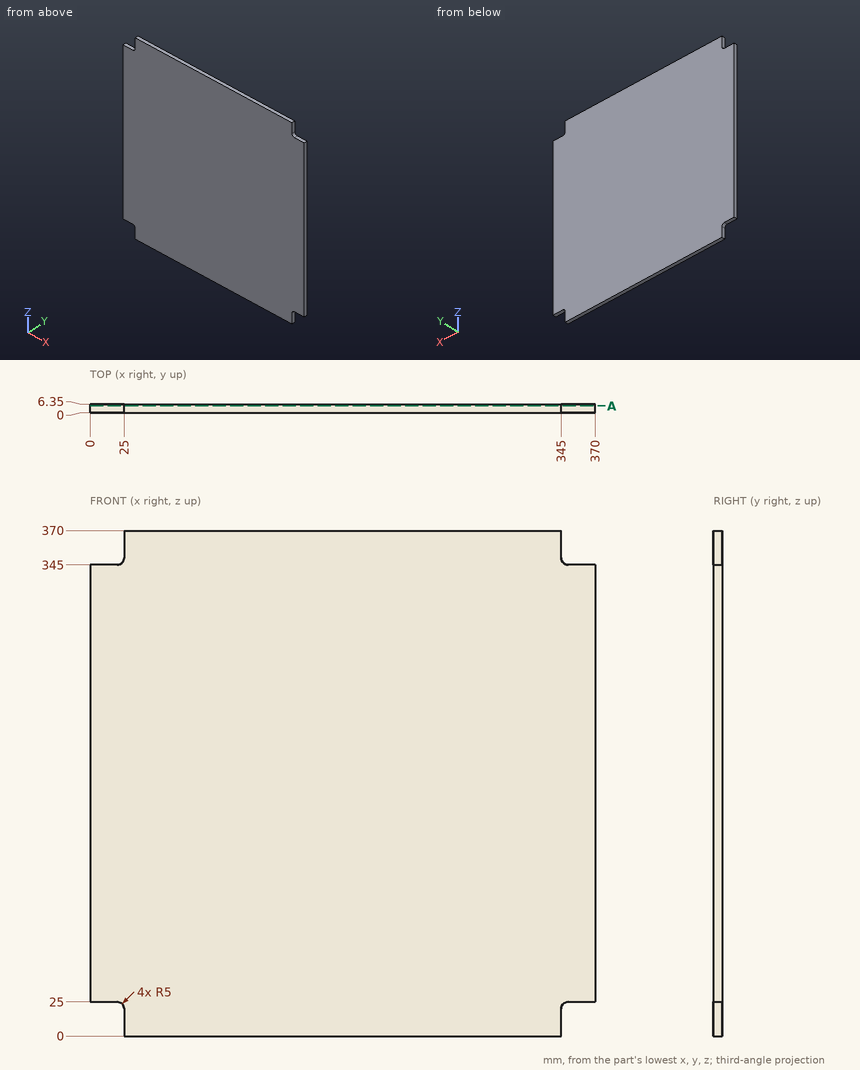
Part print with two shaded views. Sizes in mm from the minimum x, y, z corner. Give positions to 0.01 mm unless a question says otherwise; leave off trailing zeros. Order: outer loops, then holes, each group sorted by start corner. A loop starts at its lowest first (then second) coordinate and runs counter-clockwise, first axis right, second up.
1) Saw through at A-A, the plane y = 5. Write the cut outline in (x, z), then the cut area to 3 significant figures.
2) Wall check: probe 1 along Z at (x, y) = (18, 1.5); probe 2 along Z at (x, y) = (347.5, 0.75). Give the ranges that are in metal, low to high.
3) Pin check, flat tips, straight feed: pin 1 (1.9 mm diameter, centred on y = 3, z = 13.5, fed in from -X); pin 2 (3 mm diameter, centred on x = 8.5, y = 4, fed in from +Z); pin 3 (3 mm diameter, centred on x = 6, y = 3, fed in from -Z). Stop position of each tip, or through.
Computed:
1. outline: (0, 25) - (20, 25) arc R5 cw to (25, 20) - (25, 0) - (345, 0) - (345, 20) arc R5 cw to (350, 25) - (370, 25) - (370, 345) - (350, 345) arc R5 cw to (345, 350) - (345, 370) - (25, 370) - (25, 350) arc R5 cw to (20, 345) - (0, 345) - close
1. area: 134,000 mm2
2. probe 1: z = 25 to 345
2. probe 2: z = 24.33 to 345.67
3. pin 1: stops at x = 25
3. pin 2: stops at z = 345
3. pin 3: stops at z = 25
